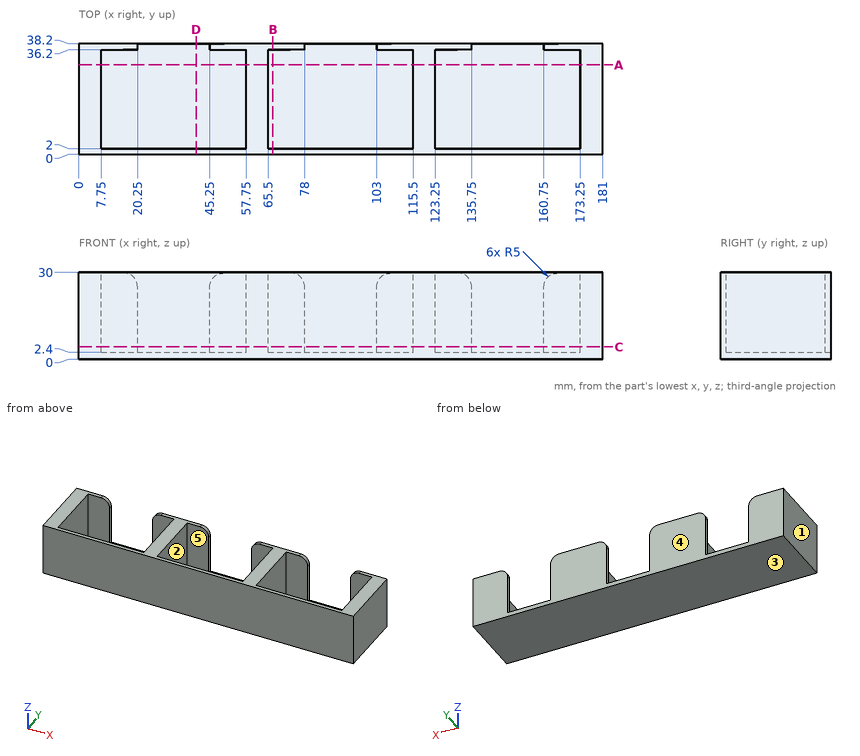
For this review, use the dimensioned drawing (mm, ordinates from the lowest corner) and the shaded views. A direction names the side the tool comes from. Give positions to 0.01 mm unless a question says otherwise; leave off trailing zeros. Order: outer loops, then holes, each group sorted by start corner. A loop starts at its lowest first (then second) coordinate and runs counter-clockwise, first axis right, second up. Notation, with made-up numbers: (36, 9) - (83, 9) arc R26 cw to (83, 37) - close; hole circle Ø5 at (7, 75.25). An arc over 180 degrees is marked (long way). Use CSV: the item, a comma, the result in double quotes. Start each with the question number.
Q1. For P1, Ø10, axis at x = 113.5, z = 18.5, coming from the -Y side; P2, Ø10, axis at x = 22.5, y = 27, coming from the +Z side; P3, Ø5, axis at x = 152, z = 6.5, coming from the +Y side, all flat-tipped, find the tip position at first contact; note any pin that passes through.
Q2. Take a section at D-D (x = 40.5). State the section outline as (y, z) points.
Q3. Take a section at A-A (y = 31). State the section outline as (x, z) points.
Q4. Take a section at B-B (x = 67). State the section outline as (y, z) points.
Q5. Take a section at C-C (z = 4.25). State the section outline as (x, y) points.
Q6. For line 1 (X direction, y = 22, z = 8.5); line 2 (Y direction, x = 53, z = 14.75); line 3 (Y direction, x = 137, z = 26.5), list the stretches that pass through material, from the lowest coordinate up.
Q7. Machinability: for the marked faces 4 and 5, which of the approach directions +Z, -Z, +X, -X, +Y, -Y give a long, thin tool a straight path to every point of the face, cutting with its end or side? Answer none if there is none.
Q8. Draft analysis for pull direction X (two halves, no side actions). For the marked faces 1, 2 and 3, state which applies: pulls with the +X half, pulls with the -X half, needs draft (parallel to the pull), parting line crosses it, or undercut.
Calculated:
1,P1,"stops at y = 0"
1,P2,"stops at z = 2.4"
1,P3,"stops at y = 2"
2,outline,"(0, 0) - (38.2, 0) - (38.2, 2.4) - (2, 2.4) - (2, 30) - (0, 30) - close"
3,outline,"(0, 0) - (181, 0) - (181, 30) - (173.25, 30) - (173.25, 2.4) - (123.25, 2.4) - (123.25, 30) - (115.5, 30) - (115.5, 2.4) - (65.5, 2.4) - (65.5, 30) - (57.75, 30) - (57.75, 2.4) - (7.75, 2.4) - (7.75, 30) - (0, 30) - close"
4,outline,"(0, 0) - (38.2, 0) - (38.2, 30) - (36.2, 30) - (36.2, 2.4) - (2, 2.4) - (2, 30) - (0, 30) - close"
5,outline,"(0, 0) - (181, 0) - (181, 38.2) - (160.75, 38.2) - (160.75, 36.2) - (173.25, 36.2) - (173.25, 2) - (123.25, 2) - (123.25, 36.2) - (135.75, 36.2) - (135.75, 38.2) - (103, 38.2) - (103, 36.2) - (115.5, 36.2) - (115.5, 2) - (65.5, 2) - (65.5, 36.2) - (78, 36.2) - (78, 38.2) - (45.25, 38.2) - (45.25, 36.2) - (57.75, 36.2) - (57.75, 2) - (7.75, 2) - (7.75, 36.2) - (20.25, 36.2) - (20.25, 38.2) - (0, 38.2) - close"
6,line 1,"x = 0 to 7.75, 57.75 to 65.5, 115.5 to 123.25, 173.25 to 181"
6,line 2,"y = 0 to 2, 36.2 to 38.2"
6,line 3,"y = 0 to 2"
7,face 4,"+Z, -Z, +X, -X, +Y"
7,face 5,"+Z"
8,face 1,"pulls with the -X half"
8,face 2,"undercut"
8,face 3,"needs draft"
